Drawing for the job (mm, zero at the part's lowest x, y, z). A direction names the side the tool comes from. Give positions to 0.01 mm unless a question says otherwise; leave off trailing zeros. Write each loop counter-clockwise with the first axis right and the second up, starting at its lowest first coordinate (ties: lowest second). Pieces come first, ordered by that corner, then holes. Notation, with made-up numbers: M -14.75,1 L -9.75,1 A21 cw -9.75,24 Z; hole C 58,7 d4. An arc over 180 degrees is marked long. Answer as a JSON object with one key per item and string values. Group by question number.
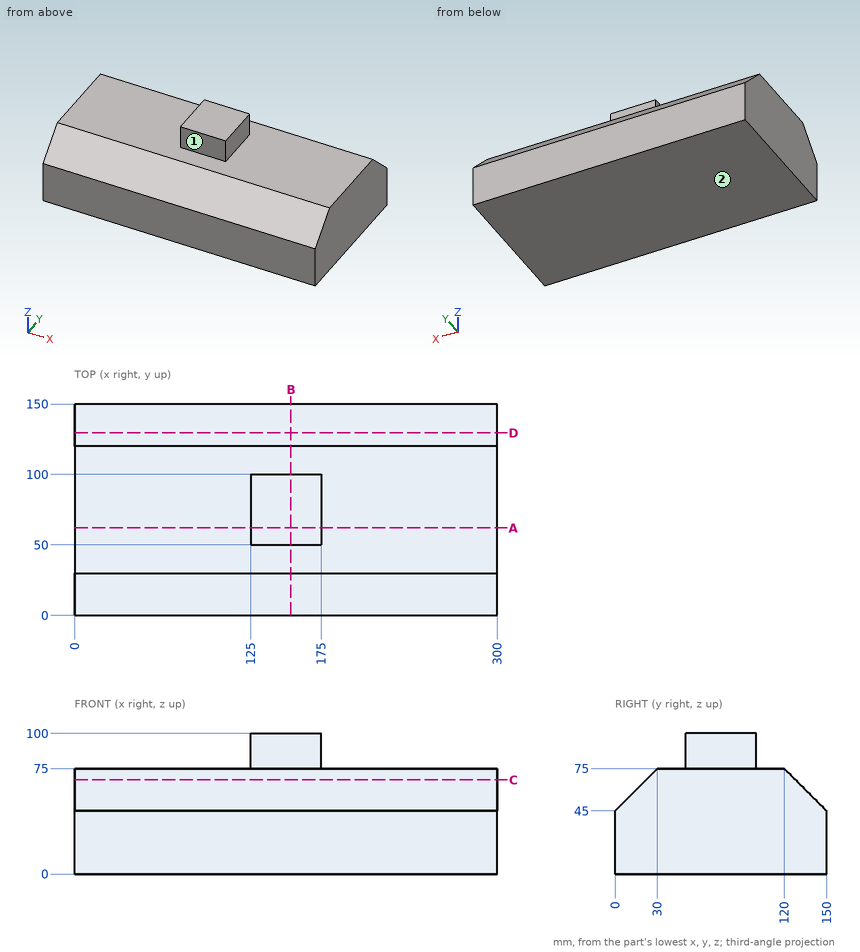
Q1. Drop flat-ended pins along their axis: P1, Ø1, axis at x = 178.5, z = 58.5, coming from the +Y side; P2, Ø20, axis at y = 87.5, z = 85.5, coming from the +X side; P3, Ø12.5, axis at x = 139, z = 86.5, coming from the +Y side. Give the stop position or say it passes through.
Q2. Slice it at D-D, the plane y = 129.5. Write the cut outline in (x, z).
Q3. Slice it at A-A, the plane y = 62. Write the cut outline in (x, z).
Q4. Slice it at C-C, the plane z = 67. Write the cut outline in (x, y), then the cut area to 3 significant figures.
Q5. Slice it at B-B, the plane x = 153.5. Write the cut outline in (y, z), then the cut area to 3 significant figures.
Q6. Wall check: L1, parallel to Z at x = 277, y = 49; L2, parallel to X at y = 74.5, z = 90.5; L3, parallel to Y at x = 110, z = 64. Give the ranges that are in metal, low to high.
Q7. 3-axis set-ups, long thin cutter, end or side, ignore diameter. For the marked faces 1 and 2: which of +Z, -Z, +X, -X, +Y, -Y reach the whole face in a straight line?
Solved:
{
 "1": {"P1": "stops at y = 137", "P2": "stops at x = 175", "P3": "stops at y = 100"},
 "2": {"outline": "M 0,0 L 300,0 L 300,65.5 L 0,65.5 Z"},
 "3": {"outline": "M 0,0 L 300,0 L 300,75 L 175,75 L 175,100 L 125,100 L 125,75 L 0,75 Z"},
 "4": {"outline": "M 0,22 L 300,22 L 300,128 L 0,128 Z", "area": "31,800 mm²"},
 "5": {"outline": "M 0,0 L 150,0 L 150,45 L 120,75 L 100,75 L 100,100 L 50,100 L 50,75 L 30,75 L 0,45 Z", "area": "11,600 mm²"},
 "6": {"L1": "z = 0 to 75", "L2": "x = 125 to 175", "L3": "y = 19 to 131"},
 "7": {"face 1": "+Z, +X, -X, -Y", "face 2": "-Z, +X, -X, +Y, -Y"}
}
